Autodesk Fusion 360 part; units mm, degrees
sketch "Sketch1" plane through (0, 0, 0) normal (0, 0, 1) x (1, 0, 0)
  circle A0 centre (0, 0) radius 65.25
  circle A1 centre (0, 0) radius 74.419 construction
  circle A2 centre (0, 74.419) radius 1.5
  circle A3 centre (-64.4487, -37.2095) radius 1.5
  circle A4 centre (64.4487, -37.2095) radius 1.5
  circle A5 centre (0, 0) radius 80
  line L0 (-80, 0) -> (80, 0) construction
  line L1 (-80, 0) -> (-80, -82.6748)
  line L2 (80, -82.6748) -> (80, 0)
  line L3 (-80, -92.6748) -> (-100, -92.6748) construction
  line L4 (-100, -92.6748) -> (-90, -92.6748)
  line L5 (100, -92.6748) -> (100, -102.6748)
  line L6 (100, -102.6748) -> (-100, -102.6748)
  line L7 (-100, -102.6748) -> (-100, -92.6748)
  arc A6 (-90, -92.6748) -> (-80, -82.6748) centre (-90, -82.6748) ccw
  line L8 (90, -92.6748) -> (100, -92.6748)
  arc A7 (80, -82.6748) -> (90, -92.6748) centre (90, -82.6748) ccw
  dimension "d1" = 130.5
  dimension "d4" = 148.838
  dimension "d5" = 3
  dimension "d7" = 360
  dimension "d8" = 160
  dimension "d10" = 200
  dimension "d11" = 10
  dimension "d12" = 10
  dimension "d13" = 10
extrude "Extrude1" add sketch "Sketch1" along normal blind 10
hole "Hole1" at (-95, -92.6748, 5) direction (0, -1, 0) diameter 5 depth 10 tip angle 118
hole "Hole2" at (95.1862, -92.6748, 5.0204) direction (0, -1, 0) diameter 5 depth 10 tip angle 118
equation "d1 = GearboxDia + Tollerance"
equation "GearboxDia = 130 mm"
equation "Tollerance = 0.5 mm"
equation "d4 = ( 74.419 * 2 ) * 1 mm"
equation "d8 = GearboxDia + 30 mm"
equation "d10 = d8 + 40 mm"
Source: CAD feature listing. Evaluate the final solid. Frame: model axes, mm. A direction names the side the tool comes from. Round coordinates to 2 decimals unless told otherwise and drop trailing zeros. Loops run counter-clockwise (first coordinate to the right, second up) from the corner with the lowest first, then second, coordinate; pieces in that order, holes last.
1. Contact query for flat-ended pins moving along their axis: pin 1 (3 mm diameter, centred on y = -11.5, z = 3.5, fed in from +X); pin 2 (2 mm diameter, centred on x = 46.5, z = 1, fed in from +Y); pin 3 (3 mm diameter, centred on x = 96, z = 3.5, fed in from +Y). Output: stop coordinate, or through.
2. Section query B-B on z = 4.25. Output: boundary loops of the cut face in (x, y).
3. Access query for faces 1 (the cylindrical face through (92.71, -97.74, 4.69)), 2 (the flat face through (-80, -41, 5)), 3 (the flat face through (80, -42, 5)). Directions: +Z, -Z, +X, -X, +Y, -Y. A direction counts if a zero-diameter tool reaches every point of the face in a straight line with its end or side. Return the directions, or none.
4. Mould query, pull axis Y, two halves, no side actions, for faces 4 (the flat face through (1, -102.675, 5)), 5 (the flat face through (-1, -71, 10)), 6 (the flat face through (92.7, -92.675, 3.8)), 7 (the cylindrical face through (62.237, -19.599, 4.93)). Classes: released by +Y, released by -Y, zero draft, split by the parting line, or undercut.
5. Section query D-D on x = 76. Output: boundary loops of the cut face in (y, z), and give its area (3 significant figures).
6. Section query A-A on x = -95. Output: boundary loops of the cut face in (y, z).
7. Section query C-C on y = -21. Output: boundary loops of the cut face in (x, z).
8. Ray query, L1, parallel to Y at x = 0, z = 7; L2, parallel to Y at x = 91.5, z = 8.5; L3, parallel to Y at x = 29, z = 4. Return the intervals inside material, ascending.
Answers below:
1. pin 1: stops at x = 80
1. pin 2: stops at y = 65.8
1. pin 3: stops at y = -92.67
2. outline: (-100, -102.67) - (-97.38, -102.67) - (-97.38, -92.67) - (-100, -92.67) - close; (-92.62, -102.67) - (92.81, -102.67) - (92.81, -92.67) - (90, -92.67) arc R10 cw to (80, -82.67) - (80, 0) arc R80 ccw to (-80, 0) - (-80, -82.67) arc R10 cw to (-90, -92.67) - (-92.62, -92.67) - close; (97.56, -102.67) - (100, -102.67) - (100, -92.67) - (97.56, -92.67) - close; hole circle Ø3 at (-64.45, -37.21); hole circle Ø130.5 at (0, 0); hole circle Ø3 at (0, 74.42); hole circle Ø3 at (64.45, -37.21)
3. face 1: +Y, -Y
3. face 2: +Z, -Z, -X, +Y
3. face 3: +Z, -Z, +X, +Y
4. face 4: released by -Y
4. face 5: zero draft
4. face 6: released by +Y
4. face 7: undercut
5. outline: (-102.67, 0) - (24.98, 0) - (24.98, 10) - (-102.67, 10) - close
5. area: 1,280 mm2
6. outline: (-102.67, 0) - (-92.67, 0) - (-92.67, 2.5) - (-102.67, 2.5) - close; (-102.67, 7.5) - (-92.67, 7.5) - (-92.67, 10) - (-102.67, 10) - close
7. outline: (-80, 0) - (-61.78, 0) - (-61.78, 10) - (-80, 10) - close; (61.78, 0) - (80, 0) - (80, 10) - (61.78, 10) - close
8. L1: y = -102.67 to -65.25, 65.25 to 72.92, 75.92 to 80
8. L2: y = -102.67 to -92.67
8. L3: y = -102.67 to -58.45, 58.45 to 74.56
